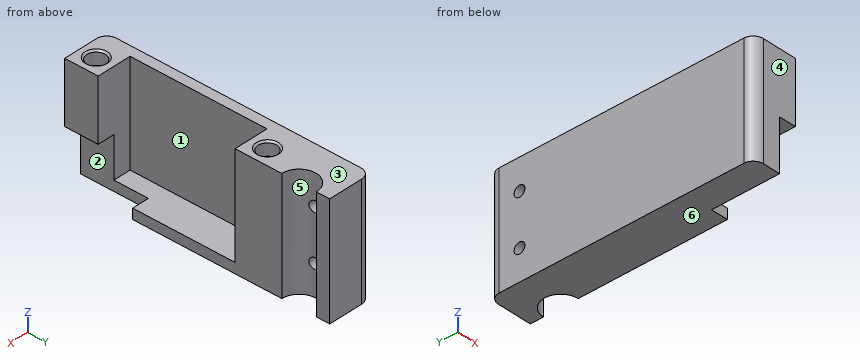
```python
from build123d import *

# Parameters (mm, degrees)
SKETCH1_W           = 26.3
SKETCH1_H           = 60
SKETCH1_W_2         = 20.3
SKETCH1_H_2         = 40.3
BOSS_EXTRUDE1_DEPTH = 30
BOSS_EXTRUDE2_START = -30
SKETCH1_2_W         = 26.3
SKETCH1_2_H         = 60
BOSS_EXTRUDE2_DEPTH = 3
SKETCH2_W           = 26.3
SKETCH2_H           = 18
SKETCH2_R           = 5.1
BOSS_EXTRUDE3_DEPTH = 33
SKETCH3_W           = 10
SKETCH3_H           = 15
CUT_EXTRUDE1_DEPTH  = 20
CUT_EXTRUDE2_DEPTH  = 64.911579545
FILLET1_R           = 3
SKETCH5_R           = 2.75
CUT_EXTRUDE3_DEPTH  = 4
CHAMFER1_SIZE       = 0.5


with BuildPart() as part:
    # Sketch1 → Boss-Extrude1 (new body)
    with BuildSketch(Plane.XY):
        Rectangle(SKETCH1_W, SKETCH1_H)
        Rectangle(SKETCH1_W_2, SKETCH1_H_2, mode=Mode.SUBTRACT)
    extrude(amount=-BOSS_EXTRUDE1_DEPTH)

    # Sketch1<2> → Boss-Extrude2 (add)
    with BuildSketch(Plane.XY.offset(BOSS_EXTRUDE2_START)):
        Rectangle(SKETCH1_2_W, SKETCH1_2_H)
    extrude(amount=-BOSS_EXTRUDE2_DEPTH)

    # Sketch2 → Boss-Extrude3 (add)
    with BuildSketch(Plane.XY):
        with Locations((0, 39)):
            Rectangle(SKETCH2_W, SKETCH2_H)
        with Locations((0, 39)):
            Circle(SKETCH2_R, mode=Mode.SUBTRACT)
    extrude(amount=-BOSS_EXTRUDE3_DEPTH)

    # Sketch3 → Cut-Extrude1 (cut)
    with BuildSketch(Plane.XZ.offset(30)):
        with Locations((0, -25.5)):
            Rectangle(SKETCH3_W, SKETCH3_H)
    extrude(amount=-CUT_EXTRUDE1_DEPTH, mode=Mode.SUBTRACT)

    # Sketch4 → Cut-Extrude2 (cut, through all)
    with BuildSketch(Plane(origin=(13.15, 0, 0), x_dir=(0, 0, -1), z_dir=(1, 0, 0))):
        with BuildLine():
            ThreePointArc((7.4, 39), (9, 37.4), (10.6, 39))
            Line((10.6, 39), (7.4, 39))
        make_face()
        with BuildLine():
            Line((7.4, 39), (10.6, 39))
            ThreePointArc((10.6, 39), (9, 40.6), (7.4, 39))
        make_face()
        with BuildLine():
            ThreePointArc((22.4, 39), (24, 37.4), (25.6, 39))
            Line((25.6, 39), (22.4, 39))
        make_face()
        with BuildLine():
            Line((22.4, 39), (25.6, 39))
            ThreePointArc((25.6, 39), (24, 40.6), (22.4, 39))
        make_face()
    extrude(amount=-CUT_EXTRUDE2_DEPTH, mode=Mode.SUBTRACT)

    # Fillet1
    fillet1_edges = [part.edges().sort_by_distance(p)[0] for p in [
        (-13.15, 48, -16.5),
        (13.15, 48, -16.5),
        (13.15, -30, -16.5),
        (-13.15, -30, -16.5),
    ]]
    fillet(fillet1_edges, radius=FILLET1_R)

    # Sketch5 → Cut-Extrude3 (cut)
    with BuildSketch(Plane.XY):
        with Locations((5.15, 25.2)):
            Circle(SKETCH5_R)
        with Locations((-4.85, 25.2)):
            Circle(SKETCH5_R)
        with Locations((5.15, -25.2)):
            Circle(SKETCH5_R)
        with Locations((-4.85, -25.2)):
            Circle(SKETCH5_R)
    extrude(amount=-CUT_EXTRUDE3_DEPTH, mode=Mode.SUBTRACT)

    # Chamfer1
    chamfer1_edges = [part.edges().sort_by_distance(p)[0] for p in [
        (-7.6, 25.2, 0),
        (2.4, -25.2, 0),
        (-7.6, -25.2, 0),
        (2.4, 25.2, 0),
    ]]
    chamfer(chamfer1_edges, length=CHAMFER1_SIZE)

    # SurfaceCut2
    split(bisect_by=Plane.ZY, keep=Keep.TOP)


solid = part.part
```
Here's how the part is built. I have some questions about the finished solid (model axes, mm). Face numbers are marked on the shaded views. A direction names the side the tool comes from. Round coordinates to 2 decimals unless told otherwise and drop trailing zeros. Order: outer loops, then holes, each group sorted by start corner. A loop starts at its lowest first (then second) coordinate and runs counter-clockwise, first axis right, second up. Notation, with made-up numbers: (83, 72.5) -> (113, 72.5) arc R7 cw to (113, 82.5) -> close; hole circle Ø11 at (55, 21.25). An arc over 180 degrees is marked (long way). Use a Markdown table: item, result. Add a question column.
(1) Suppose I cut it at D-D, the plane z = -24. Please give me the cut outline in (x, y).
(2) Suppose I cut it at A-A, the plane x = -9. Please give me the cut outline in (y, z).
(3) For pin 1 Ø4.5 at (x, y) = (-4.85, -25.2) entering from -Z; pin 2 Ø3 at (x, z) = (-3, -22) entering from -Y; pin 3 Ø7.5 at (y, z) = (-20, -25) entering from +X; pin 4 Ø2.5 at (y, z) = (39, -9) entering from -X, each with a flat end and sliding along its axis, tell me the tip position at first contact or that it passes through.
(4) Suppose I cut it at B-B, the plane z = -9. Please give me the cut outline in (x, y).
(5) I need wall thicknesses on line 1 along Z through (x, y) = (-6.75, 39); line 2 along Y through (x, z) = (-9.75, -9); line 3 along Y through (x, z) = (-6.75, -5). Which ranges of each line are inside material? Lowest first, please.
(6) Suppose I cut it at C-C, the plane y = -25.2. Please give me the cut outline in (x, z), and give its area (3 significant figures).
(7) If we mould it in two halves opening along Y, with no side actions, what happens to the marked faces 4, 5 and 6? For each: released by +Y, released by -Y, zero draft, split by the parting line, or undercut.
(8) For the marked faces 1, 2 and 3, which set-ups out of +Z, -Z, +X, -X, +Y, -Y let a thin tool reach every point of the face, with its end or its side?
Verdict:
| question | item | result |
|---|---|---|
| 1 | outline | (-13.15, -27) arc R3 ccw to (-10.15, -30) -> (-5, -30) -> (-5, -20.15) -> (-10.15, -20.15) -> (-10.15, 20.15) -> (0, 20.15) -> (0, 33.9) arc R5.1 cw to (-4.84, 37.4) -> (-13.15, 37.4) -> close; (-13.15, 40.6) -> (-4.84, 40.6) arc R5.1 cw to (0, 44.1) -> (0, 48) -> (-10.15, 48) arc R3 ccw to (-13.15, 45) -> close |
| 2 | outline | (-30, -33) -> (48, -33) -> (48, 0) -> (20.15, 0) -> (20.15, -30) -> (-20.15, -30) -> (-20.15, 0) -> (-30, 0) -> close; hole circle Ø3.2 at (39, -24); hole circle Ø3.2 at (39, -9) |
| 3 | pin 1 | z = -33 |
| 3 | pin 2 | y = 20.15 |
| 3 | pin 3 | x = -5 |
| 3 | pin 4 | through |
| 4 | outline | (-13.15, -27) arc R3 ccw to (-10.15, -30) -> (0, -30) -> (0, -20.15) -> (-10.15, -20.15) -> (-10.15, 20.15) -> (0, 20.15) -> (0, 33.9) arc R5.1 cw to (-4.84, 37.4) -> (-13.15, 37.4) -> close; (-13.15, 40.6) -> (-4.84, 40.6) arc R5.1 cw to (0, 44.1) -> (0, 48) -> (-10.15, 48) arc R3 ccw to (-13.15, 45) -> close |
| 5 | line 1 | -33 to -25.6, -22.4 to -10.6, -7.4 to 0 |
| 5 | line 2 | -30 to -20.15, 20.15 to 37.4, 40.6 to 48 |
| 5 | line 3 | -30 to -20.15, 20.15 to 48 |
| 6 | outline | (-13.15, -33) -> (-5, -33) -> (-5, -18) -> (0, -18) -> (0, 0) -> (-1.6, 0) -> (-2.1, -0.5) -> (-2.1, -4) -> (-7.6, -4) -> (-7.6, -0.5) -> (-8.1, 0) -> (-13.15, 0) -> close |
| 6 | area | 337 mm2 |
| 7 | face 4 | released by -Y |
| 7 | face 5 | undercut |
| 7 | face 6 | zero draft |
| 8 | face 1 | +Z, +X |
| 8 | face 2 | -Z, +X, -Y |
| 8 | face 3 | +Z, +X, -X, +Y, -Y |
